```python
from build123d import *

# Parameters (mm, degrees)
BASE_EXTRUDE_THIN_DEPTH = 14.097
CUT_EXTRUDE1_DEPTH      = 46.847
CUT_EXTRUDE2_DEPTH      = 1.016
CUT_EXTRUDE3_DEPTH      = 1.016


with BuildPart() as part:
    # Sketch1 → Base-Extrude-Thin (new body, symmetric)
    with BuildSketch(Plane(origin=(0, 0, 0), x_dir=(1, 0, 0), z_dir=(0, 1, 0))):
        with BuildLine():
            Line((20.6375, 0), (20.6375, 7.112))
            ThreePointArc((20.6375, 7.112), (19.670366591, 9.446866591), (17.3355, 10.414))
            Line((17.3355, 10.414), (-17.3355, 10.414))
            ThreePointArc((-17.3355, 10.414), (-19.670366591, 9.446866591), (-20.6375, 7.112))
            Line((-20.6375, 7.112), (-20.6375, 0))
            Line((-20.6375, 0), (-22.9235, 0))
            Line((-22.9235, 0), (-22.9235, 7.112))
            ThreePointArc((-22.9235, 7.112), (-21.286812693, 11.063312693), (-17.3355, 12.7))
            Line((-17.3355, 12.7), (17.3355, 12.7))
            ThreePointArc((17.3355, 12.7), (21.286812693, 11.063312693), (22.9235, 7.112))
            Line((22.9235, 7.112), (22.9235, 0))
            Line((22.9235, 0), (20.6375, 0))
        make_face()
    extrude(amount=BASE_EXTRUDE_THIN_DEPTH, both=True)

    # Sketch2 → Cut-Extrude1 (cut, through all)
    with BuildSketch(Plane(origin=(22.9235, 0, 0), x_dir=(0, 0, -1), z_dir=(1, 0, 0))):
        with BuildLine():
            Line((73.891155103, 43.867726973), (10.414, 14.097))
            Line((10.414, 14.097), (0.292293676, 9.349929105))
            ThreePointArc((0.292293676, 9.349929105), (0.079256013, 9.162474941), (0, 8.89))
            Line((0, 8.89), (0, -8.89))
            ThreePointArc((0, -8.89), (0.079256013, -9.162474941), (0.292293676, -9.349929105))
            Line((0.292293676, -9.349929105), (10.414, -14.097))
            Line((10.414, -14.097), (73.891155103, -43.867726973))
            Line((73.891155103, -43.867726973), (-66.33217255, -43.867726973))
            Line((-66.33217255, -43.867726973), (-66.33217255, 43.867726973))
            Line((-66.33217255, 43.867726973), (73.891155103, 43.867726973))
        make_face()
    extrude(amount=-CUT_EXTRUDE1_DEPTH, mode=Mode.SUBTRACT)

    # Sketch4 → Cut-Extrude2 (cut)
    with BuildSketch(Plane(origin=(22.9235, 0, 0), x_dir=(0, 0, -1), z_dir=(1, 0, 0))):
        with BuildLine():
            Line((0, 7.9375), (8.951028719, 6.854320826))
            ThreePointArc((8.951028719, 6.854320826), (9.270175347, 6.686943178), (9.398, 6.35))
            Line((9.398, 6.35), (9.398, -6.35))
            ThreePointArc((9.398, -6.35), (9.270175347, -6.686943178), (8.951028719, -6.854320826))
            Line((8.951028719, -6.854320826), (0, -7.9375))
            Line((0, -7.9375), (0, 7.9375))
        make_face()
    extrude(amount=-CUT_EXTRUDE2_DEPTH, mode=Mode.SUBTRACT)

    # Sketch5 → Cut-Extrude3 (cut)
    with BuildSketch(Plane.ZY.offset(22.9235)):
        with BuildLine():
            Line((0, 7.9375), (0, -7.9375))
            Line((0, -7.9375), (-8.951028719, -6.854320826))
            ThreePointArc((-8.951028719, -6.854320826), (-9.270175347, -6.686943178), (-9.398, -6.35))
            Line((-9.398, -6.35), (-9.398, 6.35))
            ThreePointArc((-9.398, 6.35), (-9.270175347, 6.686943178), (-8.951028719, 6.854320826))
            Line((-8.951028719, 6.854320826), (0, 7.9375))
        make_face()
    extrude(amount=-CUT_EXTRUDE3_DEPTH, mode=Mode.SUBTRACT)


solid = part.part
```
The listing builds one solid part. Answer for the finished solid, in the listing's coordinates (mm). A direction names the side the tool comes from. Give positions to 0.01 mm unless a question says otherwise; leave off trailing zeros. Order: outer loops, then holes, each group sorted by start corner. A loop starts at its lowest first (then second) coordinate and runs counter-clockwise, first axis right, second up. Notation, with made-up numbers: (-11.5, 35) -> (32.5, 35) arc R8 cw to (32.5, 40) -> close; hole circle Ø11 at (77.5, -26). An arc over 180 degrees is marked (long way). One line per item, written item: value.
1) Find section C-C, the plane x = -11. Determine the outline of the cut face in (y, z), plus the area to 3 significant figures.
Reported:
outline: (-14.1, -12.7) -> (14.1, -12.7) -> (14.1, -10.41) -> (-14.1, -10.41) -> close
area: 64.5 mm^2
2) Find section B-B, the plane y = 3. Determine the outline of the cut face in (x, z), plus the area to 3 significant figures.
Reported:
outline: (-22.43, -9.4) arc R5.59 ccw to (-17.34, -12.7) -> (17.34, -12.7) arc R5.59 ccw to (22.43, -9.4) -> (21.91, -9.4) -> (21.91, 0) -> (20.64, 0) -> (20.64, -7.11) arc R3.3 cw to (17.34, -10.41) -> (-17.34, -10.41) arc R3.3 cw to (-20.64, -7.11) -> (-20.64, 0) -> (-21.91, 0) -> (-21.91, -9.4) -> close
area: 125 mm^2
3) Flat-ended cylindrical pins translate along their axes: P1, Ø4, axis at x = 17, z = -2, coming from the -Y side; P2, Ø2, axis at y = 3, z = -5, coming from the -X side; P3, Ø2, axis at y = -2.5, z = -3.5, coming from the +X side; P4, Ø0.6, axis at x = 22.5, y = 1, coming from the +Z side. Find the tip coordinate at first contact, or state that the pin passes through.
Reported:
P1: passes through
P2: stops at x = -21.91
P3: stops at x = 21.91
P4: stops at z = -9.4
4) Find section A-A, the plane z = -5.75. Determine the outline of the cut face in (x, y).
Reported:
outline: (-22.92, -11.91) -> (-20.64, -11.91) -> (-20.64, 11.91) -> (-22.92, 11.91) -> (-22.92, 7.24) -> (-21.91, 7.24) -> (-21.91, -7.24) -> (-22.92, -7.24) -> close; (20.64, -11.91) -> (22.92, -11.91) -> (22.92, -7.24) -> (21.91, -7.24) -> (21.91, 7.24) -> (22.92, 7.24) -> (22.92, 11.91) -> (20.64, 11.91) -> close
5) Determine the mould class of faces 1 (the flat face through (21.4, -11.7, -5.3)), 2 (the flat face through (0, 0, -12.7)), 3 (the flat face through (22.423, 7.403, -4.413)) for opening direction Y: pulls with the +Y half, pulls with the -Y half, needs draft (parallel to the pull), parting line crosses it, or undercut.
Reported:
face 1: pulls with the -Y half
face 2: needs draft
face 3: undercut
6) Find the intervals of material crossed by line 1 (X direction, y = 9.5, z = -3.25); line 2 (X direction, y = -5, z = -3.25); line 3 (Z direction, x = 3, y = 11), in increasing order.
Reported:
line 1: x = -22.92 to -20.64, 20.64 to 22.92
line 2: x = -21.91 to -20.64, 20.64 to 21.91
line 3: z = -12.7 to -10.41
7) Find section D-D, the plane z = -1.5. Determine the outline of the cut face in (x, y).
Reported:
outline: (-22.92, -9.92) -> (-20.64, -9.92) -> (-20.64, 9.92) -> (-22.92, 9.92) -> (-22.92, 7.76) -> (-21.91, 7.76) -> (-21.91, -7.76) -> (-22.92, -7.76) -> close; (20.64, -9.92) -> (22.92, -9.92) -> (22.92, -7.76) -> (21.91, -7.76) -> (21.91, 7.76) -> (22.92, 7.76) -> (22.92, 9.92) -> (20.64, 9.92) -> close
8) A tool of negligible diameter and unlimited length cuts with its end or side. For faces 4 (the flat face through (21.908, 0, -5)), 5 (the flat face through (0, 0, -10.414)), 6 (the cylindrical face through (-20.591, 0.197, -11.654)), 7 (the flat face through (-21, 0, 0)), 8 (the flat face through (-22.423, -7.403, -4.413)), from which of +Z, -Z, +X, -X, +Y, -Y can it reach the whole face along a straight path? Write none if from no direction.
Reported:
face 4: +Z, +X
face 5: +Z, +Y, -Y
face 6: -Z, -X, +Y, -Y
face 7: +Z, +X, -X, +Y, -Y
face 8: +Z, -X
